Can you work these out from the model? Positions are in its coordinate system, mm. Face numbers are marked on the shaded views. A direction names the side the tool comes from. Round coordinates to 2 decimals unless told otherwise and drop trailing zeros. Order: outer loops, then holes, each group sorted by start corner. A loop starts at its lowest first (then second) coordinate and runs counter-clockwise, first axis right, second up.
Q1. For the marked faces 4, 5, 6, 7 and 8, which set-ups out of +Z, -Z, +X, -X, +Y, -Y let a thin tool reach every point of the face, with its end or its side?
Q2. If we section it at A-A (z = 6.75): Please give me the cut outline in (x, y), plus the area to 3 significant figures.
Q3. Will these pins go through, and if not, where does the flat tip stop? P1, Ø1, axis at x = 6.5, y = 0.5, coming from the +Z side; P2, Ø3, axis at y = 0.5, z = 6, coming from the +X side.
Q4. If we section it at B-B (y = 0): Please give me the cut outline in (x, z), plus the area to 3 significant figures.
Q5. If we section it at C-C (x = -3.5): Please give me the cut outline in (y, z).
Q6. If we section it at D-D (z = 1.5): Please give me the cut outline in (x, y).
Q7. We'd pull the mould along X, two halves only. Please class the marked faces 1, 2 and 3: pulls with the +X half, pulls with the -X half, needs draft (parallel to the pull), parting line crosses it, or undercut.
Q8. If I drill on line 1 (Y direction, x = 2, z = 6.25); line 2 (X direction, y = -0.2, z = 5); line 3 (X direction, y = -1.2, z = 3.5), over which ranges is the centre line in solid material (lowest first)?
from build123d import *

# Parameters (mm, degrees)
F0_W     = 14
F0_H     = 6
F0_W_2   = 8.5
F0_H_2   = 1.2
F1_DEPTH = 8
F2_W     = 4
F2_H     = 6
F3_DEPTH = 6
F4_R     = 1
F5_DEPTH = 5
F6_R     = 1


with BuildPart() as f1:
    # F0 (on Top) → F1 (new body)
    with BuildSketch(Plane.XY):
        with Locations((2, 0)):
            Rectangle(F0_W, F0_H)
        Rectangle(F0_W_2, F0_H_2, mode=Mode.SUBTRACT)
    extrude(amount=F1_DEPTH)

    # F2 (on face) → F3 (cut)
    with BuildSketch(Plane.XY.offset(8)):
        with Locations((7, 0)):
            Rectangle(F2_W, F2_H)
    extrude(amount=-F3_DEPTH, mode=Mode.SUBTRACT)

    # F4 (on face) → F5 (join)
    with BuildSketch(Plane.XY.offset(2)):
        with Locations((7, 0)):
            Circle(F4_R)
    extrude(amount=F5_DEPTH)

    # F6
    f6_edges = [f1.edges().sort_by_distance(p)[0] for p in [
        (5, 3, 5),
        (5, -3, 5),
        (9, -3, 1),
        (9, 3, 1),
        (-5, 3, 4),
        (-5, -3, 4),
    ]]
    fillet(f6_edges, radius=F6_R)


solid = f1.part
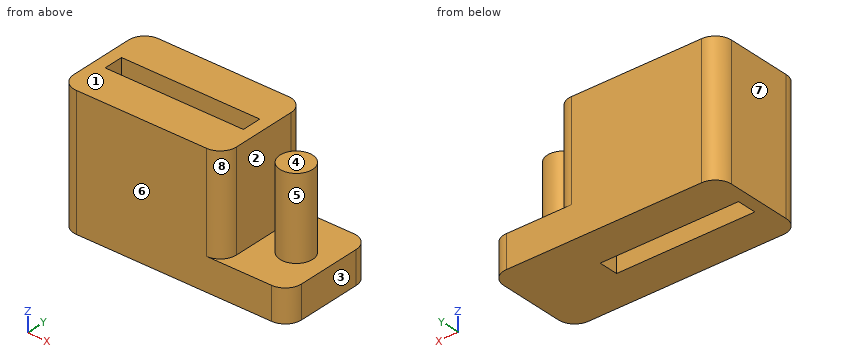
Solution:
1. face 4: +Z, +X, +Y, -Y
1. face 5: +Z
1. face 6: +Z, -Z, +X, -X, -Y
1. face 7: +Z, -Z, -X, +Y, -Y
1. face 8: +Z, +X, -Y
2. outline: (-5, -2) arc R1 ccw to (-4, -3) - (4, -3) arc R1 ccw to (5, -2) - (5, 2) arc R1 ccw to (4, 3) - (-4, 3) arc R1 ccw to (-5, 2) - close; circle Ø2 at (7, 0); hole (-4.25, -0.6) - (4.25, -0.6) - (4.25, 0.6) - (-4.25, 0.6) - close
2. area: 52.1 mm2
3. P1: stops at z = 7
3. P2: stops at x = 8
4. outline: (-5, 0) - (-4.25, 0) - (-4.25, 8) - (-5, 8) - close; (4.25, 0) - (9, 0) - (9, 2) - (8, 2) - (8, 7) - (6, 7) - (6, 2) - (5, 2) - (5, 8) - (4.25, 8) - close
4. area: 30.0 mm2
5. outline: (-3, 0) - (-0.6, 0) - (-0.6, 8) - (-3, 8) - close; (0.6, 0) - (3, 0) - (3, 8) - (0.6, 8) - close
6. outline: (-5, -2) arc R1 ccw to (-4, -3) - (8, -3) arc R1 ccw to (9, -2) - (9, 2) arc R1 ccw to (8, 3) - (-4, 3) arc R1 ccw to (-5, 2) - close; hole (-4.25, -0.6) - (4.25, -0.6) - (4.25, 0.6) - (-4.25, 0.6) - close
7. face 1: needs draft
7. face 2: undercut
7. face 3: pulls with the +X half
8. line 1: y = -3 to -0.6, 0.6 to 3
8. line 2: x = -5 to -4.25, 4.25 to 5, 6.02 to 7.98
8. line 3: x = -5 to 5
